Design review of the part built by this model. Coordinates are the model's own, in mm. A direction names the side the tool comes from. Round coordinates to 2 decimals unless told otherwise and drop trailing zeros. Loops run counter-clockwise (first coordinate to the right, second up) from the corner with the lowest first, then second, coordinate; pieces in that order, holes last. Notation, with made-up numbers: (5.25, -6) - (16.25, -6) arc R13 ccw to (16.25, 19) - close; hole circle Ø2 at (1, 26). An arc over 180 degrees is marked (long way). Answer as CSV lines item,"result". Start each with the question number.
(1) Wall thickness on L1, parallel to Y at x = -1.6, z = 0.8; L2, parallel to Z at x = 1.25, y = 7.5; L3, parallel to Z at x = 0.4, y = 16.25: over which ranges is each line inside the solid? List them lowest first.
(2) For faces 1 (the cylindrical face through (-1.216, 23.565, -1.115)), 2 (the flat face through (-1.605, 10.846, -1.016)), 3 (the cylindrical face through (-1.216, -1.565, 1.115)), list the 3-axis set-ups (+Z, -Z, +X, -X, +Y, -Y) from which the entire face can be reached by the end or side of a thin tool; tool diameter is ignored.
(3) Consider section C-C (z = -1.2). Give the boundary of the cut face in (x, y) (3 decimals).
(4) Consider section A-A (y = 9.5). Give the boundary of the cut face in (x, z).
(5) Consider section B-B (x = 0). Give the boundary of the cut face in (y, z) (3 decimals).
from build123d import *

# Parameters (mm, degrees)
BOSS_EXTRUDE1_DEPTH = 22
SKETCH2_R           = 1.65
BOSS_EXTRUDE2_DEPTH = 3.175
SKETCH3_R           = 1.65
BOSS_EXTRUDE3_DEPTH = 3.175


with BuildPart() as part:
    # Sketch1 → Boss-Extrude1 (new body)
    with BuildSketch(Plane(origin=(0, 0, 0), x_dir=(1, 0, 0), z_dir=(0, 1, 0))):
        Polygon((1.0344261, -1.934759928), (2.192764297, -0.071540683), (1.158338198, 1.863219245), (-1.0344261, 1.934759928), (-2.192764297, 0.071540683), (-1.158338198, -1.863219245), align=None)
    extrude(amount=BOSS_EXTRUDE1_DEPTH)

    # Sketch2 → Boss-Extrude2 (add)
    with BuildSketch(Plane(origin=(0, 22, 0), x_dir=(1, 0, 0), z_dir=(0, 1, 0))):
        Circle(SKETCH2_R)
    extrude(amount=BOSS_EXTRUDE2_DEPTH)

    # Sketch3 → Boss-Extrude3 (add)
    with BuildSketch(Plane.XZ):
        Circle(SKETCH3_R)
    extrude(amount=BOSS_EXTRUDE3_DEPTH)


solid = part.part
Determined:
1,L1,"y = 0 to 22"
1,L2,"z = -1.69 to 1.59"
1,L3,"z = -1.89 to 1.91"
2,face 1,"+Y"
2,face 2,"-Z, -X, +Y, -Y"
2,face 3,"-Y"
3,outline,"(-1.491, 0) - (-1.132, 0) - (-1.132, -3.175) - (1.132, -3.175) - (1.132, 0) - (1.513, 0) - (1.513, 22) - (1.132, 22) - (1.132, 25.175) - (-1.132, 25.175) - (-1.132, 22) - (-1.491, 22) - close"
4,outline,"(-2.19, -0.07) - (-1.03, -1.93) - (1.16, -1.86) - (2.19, 0.07) - (1.03, 1.93) - (-1.16, 1.86) - close"
5,outline,"(-3.175, -1.65) - (0, -1.65) - (0, -1.901) - (22, -1.901) - (22, -1.65) - (25.175, -1.65) - (25.175, 1.65) - (22, 1.65) - (22, 1.901) - (0, 1.901) - (0, 1.65) - (-3.175, 1.65) - close"
